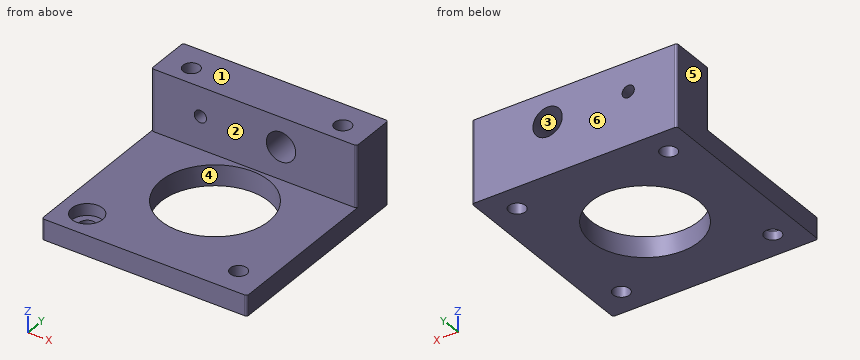
from build123d import *

# Parameters (mm, degrees)
SKETCH1_W            = 42
SKETCH1_H            = 42
BOSS_EXTRUDE1_DEPTH  = 16.8
SKETCH2_W            = 42
SKETCH2_H            = 32.65
CUT_EXTRUDE1_DEPTH   = 12.6
CUT_EXTRUDE2_REACH   = 36.121
SKETCH3_R            = 11.05
M3_CLEARANCE_HOLE1_D = 3.4
SKETCH6_R            = 3.15
CUT_EXTRUDE3_DEPTH   = 2.4
M3_TAPPED_HOLE1_D    = 2.5
FILLET1_R            = 0.5
SKETCH11_R           = 3
CUT_EXTRUDE4_DEPTH   = 10


with BuildPart() as part:
    # Sketch1 → Boss-Extrude1 (new body)
    with BuildSketch(Plane.XY):
        Rectangle(SKETCH1_W, SKETCH1_H)
    extrude(amount=BOSS_EXTRUDE1_DEPTH)

    # Sketch2 → Cut-Extrude1 (cut)
    with BuildSketch(Plane.XY.offset(16.8)):
        with Locations((0, -4.675)):
            Rectangle(SKETCH2_W, SKETCH2_H)
    extrude(amount=-CUT_EXTRUDE1_DEPTH, mode=Mode.SUBTRACT)

    # Sketch3 → Cut-Extrude2 (cut, up to next)
    with BuildSketch(Plane(origin=(0, 0, 0), x_dir=(-1, 0, 0), z_dir=(0, 0, -1)), mode=Mode.PRIVATE) as cut_extrude2_sk1:
        Circle(SKETCH3_R)
    cut_extrude2_tool1 = extrude(cut_extrude2_sk1.sketch, amount=-CUT_EXTRUDE2_REACH, mode=Mode.PRIVATE) & part.part
    add(cut_extrude2_tool1.solids().sort_by_distance((0, 0, 0))[0], mode=Mode.SUBTRACT)

    # M3 Clearance Hole1 (through all)
    with Locations(Plane.XY.offset(16.8)):
        with Locations((15.5, 15.5), (-15.5, 15.5), (-15.5, -15.5), (15.5, -15.5)):
            Hole(M3_CLEARANCE_HOLE1_D / 2)

    # Sketch6 → Cut-Extrude3 (cut)
    with BuildSketch(Plane.XY.offset(4.2)):
        with Locations((-15.5, -15.5)):
            Circle(SKETCH6_R)
    extrude(amount=-CUT_EXTRUDE3_DEPTH, mode=Mode.SUBTRACT)

    # M3 Tapped Hole1 (through all)
    with Locations(Plane(origin=(0, 21, 0), x_dir=(1, 0, 0), z_dir=(0, 1, 0))):
        with Locations((-11, -10.8)):
            Hole(M3_TAPPED_HOLE1_D / 2)

    # Fillet1
    fillet1_edges = [part.edges().sort_by_distance(p)[0] for p in [
        (21, -21, 2.1),
        (-21, -21, 2.1),
        (-21, 11.65, 10.5),
        (21, 11.65, 10.5),
        (-21, 21, 8.4),
        (21, 21, 8.4),
    ]]
    fillet(fillet1_edges, radius=FILLET1_R)

    # Sketch11 → Cut-Extrude4 (cut)
    with BuildSketch(Plane(origin=(0, 21, 0), x_dir=(1, 0, 0), z_dir=(0, 1, 0))):
        with Locations(Location((5.5, -10.8, 0), (0, 0, 270))):
            Circle(SKETCH11_R)
    extrude(amount=-CUT_EXTRUDE4_DEPTH, mode=Mode.SUBTRACT)


solid = part.part
Input: part model. Units: mm. Frame: model coordinates. Face numbers are marked on the shaded views. A direction names the side the tool comes from. Give positions to 0.01 mm unless a question says otherwise; leave off trailing zeros. Loops run counter-clockwise (first coordinate to the right, second up) from the corner with the lowest first, then second, coordinate; pieces in that order, holes last. Notation, with made-up numbers: (-2, 30) -> (9, 30) arc R5 cw to (9, 39) -> close; hole circle Ø4 at (37.25, 23.5). An arc over 180 degrees is marked (long way). Answer as a JSON object with one key per item and string values. Group by question number.
Item 1: Cut plane D-D, the plane z = 14.75. Return the cut outline in (x, y).
Item 2: Pull-direction query (X, two-part tool) for the marked faces 3, 4, 5 and 6; classes: released by +X, released by -X, zero draft, split by the parting line, or undercut.
Item 3: Cut plane A-A, the plane x = -15.5. Return the cut outline in (y, z).
Item 4: Cut plane B-B, the plane z = 11.5. Return the cut outline in (x, y).
Item 5: Reachability of the marked faces 1 and 2 from +Z, -Z, +X, -X, +Y, -Y: full face, straight path, thin tool, end or side. Return the list, or none.
Item 6: Pin query (flat end, axial travel): P1, Ø8, axis at x = 2.5, z = 14.5, coming from the -Y side; P2, Ø20, axis at x = 0, y = 0, coming from the -Z side; P3, Ø3, axis at x = -2, y = -11.5, coming from the +Z side; P4, Ø1.9, axis at x = -14.5, y = -16, coming from the +Z side. Return the tip coordinate at first contact, or that it passes through.
Item 7: Cut plane C-C, the plane y = 15. Return the cut outline in (x, z), and give its area (3 significant figures).
Item 8: Line query: probe 1 along X at (y, z) = (17.75, 10.8); probe 2 along X at (y, z) = (16, 10.8); probe 3 along Y at (x, z) = (11, 5.5). Output: solid intervals per line, ascending.
Checks:
{
 "1": {"outline": "(-21, 12.15) arc R0.5 ccw to (-20.5, 11.65) -> (20.5, 11.65) arc R0.5 ccw to (21, 12.15) -> (21, 20.5) arc R0.5 ccw to (20.5, 21) -> (-20.5, 21) arc R0.5 ccw to (-21, 20.5) -> close; hole circle Ø3.4 at (-15.5, 15.5); hole circle Ø3.4 at (15.5, 15.5)"},
 "2": {"face 3": "undercut", "face 4": "undercut", "face 5": "released by -X", "face 6": "zero draft"},
 "3": {"outline": "(-21, 0) -> (-17.2, 0) -> (-17.2, 1.8) -> (-18.65, 1.8) -> (-18.65, 4.2) -> (-21, 4.2) -> close; (-13.8, 0) -> (13.8, 0) -> (13.8, 16.8) -> (11.65, 16.8) -> (11.65, 4.2) -> (-12.35, 4.2) -> (-12.35, 1.8) -> (-13.8, 1.8) -> close; (17.2, 0) -> (21, 0) -> (21, 16.8) -> (17.2, 16.8) -> close"},
 "4": {"outline": "(-21, 12.15) arc R0.5 ccw to (-20.5, 11.65) -> (-12.04, 11.65) -> (-12.04, 21) -> (-20.5, 21) arc R0.5 ccw to (-21, 20.5) -> close; (-9.96, 11.65) -> (2.58, 11.65) -> (2.58, 21) -> (-9.96, 21) -> close; (8.42, 11.65) -> (20.5, 11.65) arc R0.5 ccw to (21, 12.15) -> (21, 20.5) arc R0.5 ccw to (20.5, 21) -> (8.42, 21) -> close; hole circle Ø3.4 at (-15.5, 15.5); hole circle Ø3.4 at (15.5, 15.5)"},
 "5": {"face 1": "+Z, +X, -X, +Y, -Y", "face 2": "+Z, +X, -X, -Y"},
 "6": {"P1": "stops at y = 11.65", "P2": "passes through", "P3": "stops at z = 4.2", "P4": "stops at z = 1.8"},
 "7": {"outline": "(-21, 0) -> (-17.12, 0) -> (-17.12, 16.8) -> (-21, 16.8) -> close; (-13.88, 0) -> (13.88, 0) -> (13.88, 16.8) -> (-13.88, 16.8) -> close; (17.12, 0) -> (21, 0) -> (21, 16.8) -> (17.12, 16.8) -> close; hole circle Ø2.5 at (-11, 10.8); hole circle Ø6 at (5.5, 10.8)", "area": "563 mm²"},
 "8": {"probe 1": "x = -21 to -12.25, -9.75 to 2.5, 8.5 to 21", "probe 2": "x = -21 to -17.12, -13.88 to -12.25, -9.75 to 2.5, 8.5 to 13.88, 17.12 to 21", "probe 3": "y = 11.65 to 21"}
}
